Check sheet for the modelled part. Datum: model origin and axes. Units: mm. Face numbers are marked on the shaded views. A direction names the side the tool comes from. Coordinates: 2 decimals unless noted, no trailing zeros. Write each loop counter-clockwise with the first axis right and the second up, starting at its lowest first coordinate (ties: lowest second). Pieces come first, ordered by that corner, then holes. Notation, with made-up numbers: (-2, 61) -> (27, 61) arc R27 ccw to (27, 84) -> close; hole circle Ø6 at (-31.75, 89.25). An arc over 180 degrees is marked (long way). Put each result on its own line as item: value.
```python
from build123d import *

# Parameters (mm, degrees)
F1_DEPTH = 2
F0_W     = 13
F0_H     = 3
F2_DEPTH = 7
F3_START = 5
F3_DEPTH = 2
F4_R     = 1
F5_R     = 5


with BuildPart() as f1:
    # F0 (on Front) → F1 (new body)
    with BuildSketch(Plane.XZ):
        with BuildLine():
            Line((3.8078865529, 1.65), (4.9839743178, 1.65))
            ThreePointArc((4.9839743178, 1.65), (3.7123106012, 3.7123106012), (1.65, 4.9839743178))
            Line((1.65, 4.9839743178), (1.65, 3.8078865529))
            ThreePointArc((1.65, 3.8078865529), (2.9344931419, 2.9344931419), (3.8078865529, 1.65))
        make_face()
        with BuildLine():
            ThreePointArc((-1.65, 4.9839743178), (-3.7123106012, 3.7123106012), (-4.9839743178, 1.65))
            Line((-4.9839743178, 1.65), (-3.8078865529, 1.65))
            ThreePointArc((-3.8078865529, 1.65), (-2.9344931419, 2.9344931419), (-1.65, 3.8078865529))
            Line((-1.65, 3.8078865529), (-1.65, 4.9839743178))
        make_face()
        with BuildLine():
            Line((-3.8078865529, -1.65), (-4.9839743178, -1.65))
            ThreePointArc((-4.9839743178, -1.65), (-3.7123106012, -3.7123106012), (-1.65, -4.9839743178))
            Line((-1.65, -4.9839743178), (-1.65, -3.8078865529))
            ThreePointArc((-1.65, -3.8078865529), (-2.9344931419, -2.9344931419), (-3.8078865529, -1.65))
        make_face()
        with BuildLine():
            ThreePointArc((1.65, -4.9839743178), (3.7123106012, -3.7123106012), (4.9839743178, -1.65))
            Line((4.9839743178, -1.65), (3.8078865529, -1.65))
            ThreePointArc((3.8078865529, -1.65), (2.9344931419, -2.9344931419), (1.65, -3.8078865529))
            Line((1.65, -3.8078865529), (1.65, -4.9839743178))
        make_face()
        with BuildLine():
            Line((-5.25, 0), (-6.5, 0))
            ThreePointArc((-6.5, 0), (0, -6.5), (6.5, 0))
            Line((6.5, 0), (5.25, 0))
            ThreePointArc((5.25, 0), (5.1830669091, -0.8356538852), (4.9839743178, -1.65))
            ThreePointArc((4.9839743178, -1.65), (3.7123106012, -3.7123106012), (1.65, -4.9839743178))
            ThreePointArc((1.65, -4.9839743178), (0, -5.25), (-1.65, -4.9839743178))
            ThreePointArc((-1.65, -4.9839743178), (-3.7123106012, -3.7123106012), (-4.9839743178, -1.65))
            ThreePointArc((-4.9839743178, -1.65), (-5.1830669091, -0.8356538852), (-5.25, 0))
        make_face()
        with BuildLine():
            ThreePointArc((-2.3184322471, 6.0724683544), (-5.3534946346, 3.6864746299), (-6.5, 0))
            Line((-6.5, 0), (-5.25, 0))
            ThreePointArc((-5.25, 0), (-5.1830669091, 0.8356538852), (-4.9839743178, 1.65))
            ThreePointArc((-4.9839743178, 1.65), (-3.7123106012, 3.7123106012), (-1.65, 4.9839743178))
            ThreePointArc((-1.65, 4.9839743178), (0, 5.25), (1.65, 4.9839743178))
            ThreePointArc((1.65, 4.9839743178), (3.7123106012, 3.7123106012), (4.9839743178, 1.65))
            ThreePointArc((4.9839743178, 1.65), (5.1830669091, 0.8356538852), (5.25, 0))
            Line((5.25, 0), (6.5, 0))
            ThreePointArc((6.5, 0), (5.3534946346, 3.6864746299), (2.3184322471, 6.0724683544))
            ThreePointArc((2.3184322471, 6.0724683544), (0, 5.8), (-2.3184322471, 6.0724683544))
        make_face()
        with BuildLine():
            ThreePointArc((2.3184322471, 6.0724683544), (0, 6.5), (-2.3184322471, 6.0724683544))
            ThreePointArc((-2.3184322471, 6.0724683544), (0, 5.8), (2.3184322471, 6.0724683544))
        make_face()
        with BuildLine():
            Line((-6.5, 8.2006579232), (-6.5, 0))
            ThreePointArc((-6.5, 0), (-5.3534946346, 3.6864746299), (-2.3184322471, 6.0724683544))
            ThreePointArc((-2.3184322471, 6.0724683544), (-4.5358003191, 6.8878445107), (-6.5, 8.2006579232))
        make_face()
        with BuildLine():
            ThreePointArc((2.3184322471, 6.0724683544), (5.3534946346, 3.6864746299), (6.5, 0))
            Line((6.5, 0), (6.5, 8.2006579232))
            ThreePointArc((6.5, 8.2006579232), (4.5358003191, 6.8878445107), (2.3184322471, 6.0724683544))
        make_face()
        with BuildLine():
            ThreePointArc((-6.5, 8.2006579232), (-4.5358003191, 6.8878445107), (-2.3184322471, 6.0724683544))
            ThreePointArc((-2.3184322471, 6.0724683544), (0, 6.5), (2.3184322471, 6.0724683544))
            ThreePointArc((2.3184322471, 6.0724683544), (4.5358003191, 6.8878445107), (6.5, 8.2006579232))
            Line((6.5, 8.2006579232), (6.5, 11.5))
            Line((6.5, 11.5), (-6.5, 11.5))
            Line((-6.5, 11.5), (-6.5, 8.2006579232))
        make_face()
    extrude(amount=F1_DEPTH)

    # F0 (on Front) → F2 (join)
    with BuildSketch(Plane.XZ):
        with Locations((0, 13)):
            Rectangle(F0_W, F0_H)
    extrude(amount=F2_DEPTH)

    # F0 (on Front) → F3 (join)
    with BuildSketch(Plane.XZ.offset(F3_START)):
        with BuildLine():
            ThreePointArc((-6.3804388564, 23.5), (-6.4404160803, 23.4499046211), (-6.5, 23.3993420768))
            Line((-6.5, 23.3993420768), (-6.5, 14.5))
            Line((-6.5, 14.5), (6.5, 14.5))
            Line((6.5, 14.5), (6.5, 23.3993420768))
            ThreePointArc((6.5, 23.3993420768), (6.4404160803, 23.4499046211), (6.3804388564, 23.5))
            Line((6.3804388564, 23.5), (-6.3804388564, 23.5))
        make_face()
        with BuildLine():
            ThreePointArc((6.3804388564, 23.5), (0, 25.8), (-6.3804388564, 23.5))
            Line((-6.3804388564, 23.5), (6.3804388564, 23.5))
        make_face()
    extrude(amount=F3_DEPTH)

    # F4
    f4_edges = [f1.edges().sort_by_distance(p)[0] for p in [
        (0, -2, 11.5),
        (0, -7, 11.5),
        (0, 0, 14.5),
        (0, -5, 14.5),
    ]]
    fillet(f4_edges, radius=F4_R)

    # F5
    f5_edges = [f1.edges().sort_by_distance(p)[0] for p in [
        (6.5, -6, 23.399342),
        (-6.5, -6, 23.399342),
    ]]
    fillet(f5_edges, radius=F5_R)


solid = f1.part
```
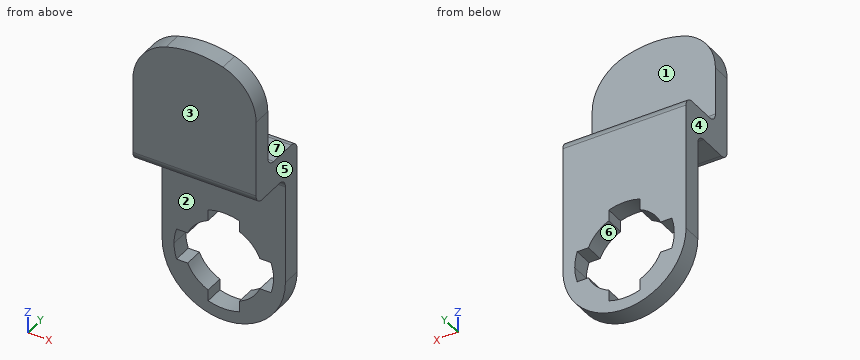
Q1. Cross-section at B-B (y = -1.5). Record the cut outline in (x, z), plus the area to 3 significant figures.
Recorded:
outline: (-6.5, 0) arc R6.5 ccw to (6.5, 0) -> (6.5, 14.5) -> (-6.5, 14.5) -> close; hole (-4.98, -1.65) -> (-3.81, -1.65) arc R4.15 ccw to (-1.65, -3.81) -> (-1.65, -4.98) arc R5.25 ccw to (1.65, -4.98) -> (1.65, -3.81) arc R4.15 ccw to (3.81, -1.65) -> (4.98, -1.65) arc R5.25 ccw to (4.98, 1.65) -> (3.81, 1.65) arc R4.15 ccw to (1.65, 3.81) -> (1.65, 4.98) arc R5.25 ccw to (-1.65, 4.98) -> (-1.65, 3.81) arc R4.15 ccw to (-3.81, 1.65) -> (-4.98, 1.65) arc R5.25 ccw to start
area: 186 mm2
Q2. Cross-section at D-D (z = 19). Record the cut outline in (x, y).
Recorded:
outline: (-6.5, -7) -> (6.5, -7) -> (6.5, -5) -> (-6.5, -5) -> close
Q3. Mould release check, pull along X, two halves, no side actions. Record for the marked faces 4, 5, 6 and 7: released by +X, released by -X, zero draft, split by the parting line, or undercut.
Recorded:
face 4: released by -X
face 5: released by +X
face 6: undercut
face 7: zero draft
Q4. Cross-section at C-C (z = -1). Record the cut outline in (x, y).
Recorded:
outline: (-6.42, -2) -> (-5.15, -2) -> (-5.15, 0) -> (-6.42, 0) -> close; (5.15, -2) -> (6.42, -2) -> (6.42, 0) -> (5.15, 0) -> close
Q5. Cross-section at A-A (x = -0.5). Record the cut outline in (y, z), plus the area to 3 significant figures.
Recorded:
outline: (-7, 12.5) arc R1 ccw to (-6, 11.5) -> (-3, 11.5) arc R1 cw to (-2, 10.5) -> (-2, 5.23) -> (0, 5.23) -> (0, 13.5) arc R1 ccw to (-1, 14.5) -> (-4, 14.5) arc R1 cw to (-5, 15.5) -> (-5, 25.79) -> (-7, 25.79) -> close; (-2, -6.48) -> (0, -6.48) -> (0, -5.23) -> (-2, -5.23) -> close
area: 58.6 mm2
Q6. Depth check by flat-ended pin: P1, Ø4, axis at x = -1, z = 21, coming from the +Y side; P2, Ø1.5, axis at y = -3.5, z = 18.5, coming from the -X side; P3, Ø1.5, axis at x = 2.5, y = -4.5, coming from the -Z side; P4, Ø1.5, axis at x = 1, z = 14.5, coming from the +Y side. Enter the tip coordinate at first touch or a pass-through.
Recorded:
P1: stops at y = -5
P2: passes through
P3: stops at z = 11.5
P4: stops at y = -0.03
Q7. Tool access check on the marked faces 1, 2 and 3. Record the directions out of +Z, -Z, +X, -X, +Y, -Y that give a thin tool (end or side, any length) a straight path to the whole face; none if there is none.
Recorded:
face 1: +Z, +X, -X, +Y
face 2: -Z, +X, -X, -Y
face 3: +Z, -Z, +X, -X, -Y
Q8. Material ranges on line 1 along Y through (x, z) = (5, 9); line 2 along Y through (x, z) = (-5.25, 20.5); line 3 along Z through (x, y) = (2.25, -3.5), recorded low to high.
Recorded:
line 1: y = -2 to 0
line 2: y = -7 to -5
line 3: z = 11.5 to 14.5
